Work out the finished part from the listing and answer in its coordinate system (mm). Face numbers are marked on the shaded views. A direction names the side the tool comes from. Coordinates: 2 decimals unless noted, no trailing zeros. Order: outer loops, then holes, each group sorted by start corner. A loop starts at its lowest first (then second) coordinate and runs counter-clockwise, first axis right, second up. Notation, with made-up numbers: (84, 69) -> (121, 69) arc R18 cw to (121, 104) -> close; hole circle Ø7 at (33, -27.5). An arc over 180 degrees is marked (long way). Answer as CSV lines item,"result". Start each with the question number.
Item 1: Straight lines are drawn through the part: L1, parallel to Z at x = -7.5, y = -9.75; L2, parallel to Y at x = -8.25, z = 10; L3, parallel to Z at x = -9, y = -4.5. For each, find the intervals that lie inside material, in ascending order.
Item 2: Section B-B (y = 1) is taken. Write down the section's boundary in (x, z), then the cut area to 3 significant figures.
Item 3: For a pull along Y with two mould halves and no side action, classify the marked faces 1, 2 and 3 as pulls with the +Y half, pulls with the -Y half, needs draft (parallel to the pull), parting line crosses it, or undercut.
Item 4: Which of the six approach directions +Z, -Z, +X, -X, +Y, -Y give full straight-line access (tool end or side, diameter ignored) to the marked faces 4, 5 and 6?
Item 5: Each of these flat-tipped pins is pushed along its axis until it touches: pin 1 Ø4 at (x, y) = (-2.5, 7) entering from +Z; pin 2 Ø1.5 at (x, z) = (-3.5, 0) entering from +Y. Where does it stop, or does it pass through?
Item 6: Section A-A (z = 0) is taken. Write down the section's boundary in (x, y).
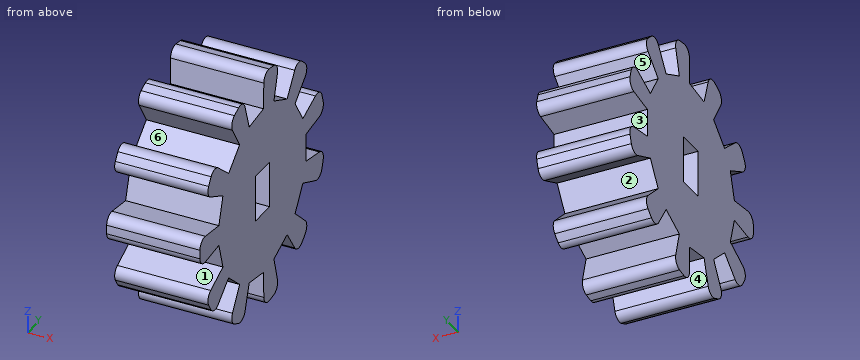
```python
from build123d import *

# Parameters (mm, degrees)
SKETCH1_W                = 10
SKETCH1_H                = 13
CUT_EXTRUDE1_DEPTH       = 10
SKETCH7_W                = 5
SKETCH7_H                = 3
CUT_EXTRUDE2_DEPTH       = 10
FILLET1_R                = 1
CIRPATTERN1_COUNT        = 11
FILLET1_OF_CIRPATTERN1_R = 1


with BuildPart() as part:
    # Sketch1 → Revolve1 (revolve)
    with BuildSketch(Plane.XY):
        with Locations((-5, 6.5)):
            Rectangle(SKETCH1_W, SKETCH1_H)
    revolve(axis=Axis((-10, 0, 0), (-1, 0, 0)))

    # Sketch6 → Cut-Extrude1 (cut)
    with BuildSketch(Plane(origin=(0, 0, 0), x_dir=(0, 0, -1), z_dir=(1, 0, 0))):
        Polygon((-1.501758676, 9), (1.501758676, 9), (2.502016427, 15), (-2.502016427, 15), align=None)
    cut_extrude1 = extrude(amount=-CUT_EXTRUDE1_DEPTH, mode=Mode.SUBTRACT)

    # Sketch7 → Cut-Extrude2 (cut)
    with BuildSketch(Plane(origin=(0, 0, 0), x_dir=(0, 0, -1), z_dir=(1, 0, 0))):
        Rectangle(SKETCH7_W, SKETCH7_H)
    extrude(amount=-CUT_EXTRUDE2_DEPTH, mode=Mode.SUBTRACT)

    # Fillet1
    fillet1_edges = [part.edges().sort_by_distance(p)[0] for p in [
        (-5, 12.822809052, 2.13905774),
        (-5, 12.822809052, -2.13905774),
    ]]
    fillet(fillet1_edges, radius=FILLET1_R)

    # CirPattern1: Cut-Extrude1 ×11 about axis
    cirpattern1_axis = Axis((0, 0, 0), (1, 0, 0))
    for i in range(1, CIRPATTERN1_COUNT):
        add(cut_extrude1.rotate(cirpattern1_axis, i * 360 / CIRPATTERN1_COUNT), mode=Mode.SUBTRACT)

    # Fillet1 of CirPattern1
    fillet1_of_cirpattern1_edges = [part.edges().sort_by_distance(p)[0] for p in [
        (-5, 9.630771491, 8.732023849),
        (-5, 11.943695341, 5.133044087),
        (-5, 3.381032029, 12.552634083),
        (-5, 7.27254275, 10.775440685),
        (-5, -3.942161213, 12.387871688),
        (-5, 0.29240922, 12.996711001),
        (-5, -10.013746124, 8.290047561),
        (-5, -6.78056217, 11.091617405),
        (-5, -12.906037394, 1.560191908),
        (-5, -11.700752981, 5.665013652),
        (-5, -11.700752981, -5.665013652),
        (-5, -12.906037394, -1.560191908),
        (-5, -6.78056217, -11.091617405),
        (-5, -10.013746124, -8.290047561),
        (-5, 0.29240922, -12.996711001),
        (-5, -3.942161213, -12.387871688),
        (-5, 7.27254275, -10.775440685),
        (-5, 3.381032029, -12.552634083),
        (-5, 11.943695341, -5.133044087),
        (-5, 9.630771491, -8.732023849),
    ]]
    fillet(fillet1_of_cirpattern1_edges, radius=FILLET1_OF_CIRPATTERN1_R)


solid = part.part
```
Checked values:
1,L1,"z = -7.85 to -4.72, -1.18 to 1.18, 4.72 to 7.85"
1,L2,"y = -6.11 to -3.18, 0.23 to 2.69, 6.76 to 8.31"
1,L3,"z = -12.09 to 12.09"
2,outline,"(-10, -12.9) -> (0, -12.9) -> (0, -2.5) -> (-10, -2.5) -> close; (-10, 2.5) -> (0, 2.5) -> (0, 12.9) -> (-10, 12.9) -> close"
2,area,"208 mm^2"
3,face 1,"pulls with the -Y half"
3,face 2,"undercut"
3,face 3,"pulls with the +Y half"
4,face 4,"-Z, +X, -X"
4,face 5,"+X, -X, +Y"
4,face 6,"+X, -X"
5,pin 1,"stops at z = 10.35"
5,pin 2,"stops at y = 9"
6,outline,"(-10, -13) -> (0, -13) -> (0, -1.5) -> (-10, -1.5) -> close; (-10, 1.5) -> (0, 1.5) -> (0, 9) -> (-10, 9) -> close"
